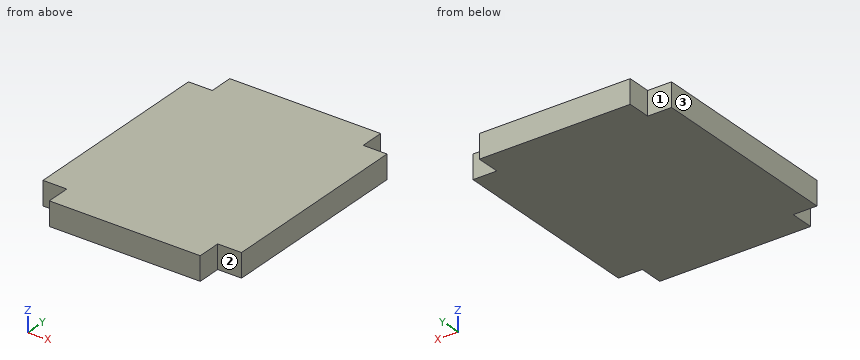
Autodesk Inventor part; units mm, degrees
ref_plane "YZ Plane" through (0, 0, 0) normal (1, 0, 0) x (0, 1, 0)
ref_plane "XZ Plane" through (0, 0, 0) normal (0, 1, 0) x (-1, 0, 0)
ref_plane "XY Plane" through (0, 0, 0) normal (0, 0, 1) x (1, 0, 0)
sketch "Sketch1" plane through (0, 0, 0) normal (0, 0, 1) x (1, 0, 0)
  line L0 (0, 0) -> (19, 0)
  line L1 (19, 0) -> (19, 31)
  line L2 (19, 31) -> (0, 31)
  line L3 (0, 31) -> (0, 0)
  line L4 (-3, 28) -> (0, 28)
  line L5 (0, 28) -> (0, 3)
  line L6 (0, 3) -> (-3, 3)
  line L7 (-3, 3) -> (-3, 28)
  line L8 (-3, 28) -> (0, 3) construction
  line L9 (0, 28) -> (-3, 3) construction
  line L10 (22, 28) -> (19, 28)
  line L11 (19, 28) -> (19, 3)
  line L12 (19, 3) -> (22, 3)
  line L13 (22, 3) -> (22, 28)
  line L14 (22, 28) -> (19, 3) construction
  line L15 (19, 28) -> (22, 3) construction
  point P0 (-1.5, 15.5)
  point P1 (20.5, 15.5)
  point P2 (0, 15.5)
  point P3 (0, 15.5)
  point P4 (0, 28)
  dimension "d0" = 19
  dimension "d1" = 31
  dimension "d2" = 3
  dimension "d3" = 3
  dimension "d4" = 25
extrude "Extrusion1" add sketch "Sketch1" along normal blind 3
properties part number "Frontrail"
Model file for the job. Use its own axes, mm. Face numbers are marked on the shaded views. A direction names the side the tool comes from. Give positions to 0.01 mm unless a question says otherwise; leave off trailing zeros. Order: outer loops, then holes, each group sorted by start corner. A loop starts at its lowest first (then second) coordinate and runs counter-clockwise, first axis right, second up. Notation, with made-up numbers: (83, 35) - (117, 35) arc R16 ccw to (117, 64) - close; hole circle Ø5 at (38, 6). An arc over 180 degrees is marked (long way). Return JSON: item names as keys, results as strings.
1) Cut at B-B, the plane y = 2.5. Give the cut face in (x, z).
Geometry says:
{"outline": "(0, 0) - (19, 0) - (19, 3) - (0, 3) - close"}
2) Flat gauge pins, fed straight in: P1, Ø0.9, axis at x = -1.5, z = 1, coming from the -Y side; P2, Ø1.5, axis at y = 29.5, z = 1.5, coming from the -X side; P3, Ø8, axis at x = 16.5, y = 21.5, coming from the -Z side; P4, Ø0.9, axis at y = 1.5, z = 1, coming from the +X side. Where does each tip first touch, or does it go through?
Geometry says:
{"P1": "y = 3", "P2": "x = 0", "P3": "z = 0", "P4": "x = 19"}
3) Cut at A-A, the plane z = 1.3. Give the cut face in (x, y), plus the area to 3 significant figures.
Geometry says:
{"outline": "(-3, 3) - (0, 3) - (0, 0) - (19, 0) - (19, 3) - (22, 3) - (22, 28) - (19, 28) - (19, 31) - (0, 31) - (0, 28) - (-3, 28) - close", "area": "739 mm²"}
4) 3-axis set-ups, long thin cutter, end or side, ignore diameter. For the marked faces 1, 2 and 3: which of +Z, -Z, +X, -X, +Y, -Y reach the whole face in a straight line?
Geometry says:
{"face 1": "+Z, -Z, -X, +Y", "face 2": "+Z, -Z, +X, -Y", "face 3": "+Z, -Z, -X, +Y, -Y"}
5) Probe line 1 (X direction, y = 2, z = 2.3). List the from-to ranges inside material, lowest first. Write a range as from..to.
Geometry says:
{"line 1": "0..19"}
